The model under review builds one solid part; all positions refer to its coordinate system, in mm. Face numbers are marked on the shaded views. Round coordinates to 2 decimals unless told otherwise and drop trailing zeros. Write each loop counter-clockwise with the first axis right and the second up, starting at its lowest first coordinate (ties: lowest second). Pieces come first, ordered by that corner, then holes. Notation, with made-up numbers: (41.5, -23) -> (54.5, -23) arc R27 cw to (54.5, 16) -> close; hole circle Ø8 at (46, -16.75). An arc over 180 degrees is marked (long way). Return JSON: item names as keys, results as strings. Group by question number.
1. Take a section at B-B, the plane x = 7. Write out the cut boundary in (y, z), then the cut area to 3 significant figures.
2. Mouldability with a two-part tool opening along X and no side actions: class the marked faces 1, 2, 3 and 4 as pulls with the +X half, pulls with the -X half, needs draft (parallel to the pull), parting line crosses it, or undercut.
3. For line 1 along Y through (x, z) = (1.5, 1.15); line 2 along X through (y, z) = (10, 2.6); line 3 along Y through (x, z) = (14, 2.75), list the stretches that pass through material, from the lowest coordinate up. Write a range as from..to.
4. Take a section at A-A, the plane z = 1.35. Write out the cut boundary in (x, y), then the cut area to 3 significant figures.
5. Take a section at D-D, the plane y = -10. Write out the cut boundary in (x, z).
6. Clearance check with flat-ended pins moving along their axes: P1, Ø12, axis at x = 8.5, y = -11, coming from the -Z side; P2, Ø1.5, axis at x = 2, z = 1.5, coming from the -Y side. State where each tip first meets the part, or that it passes through.
7. Take a section at C-C, the plane y = 10. Write out the cut boundary in (x, z).
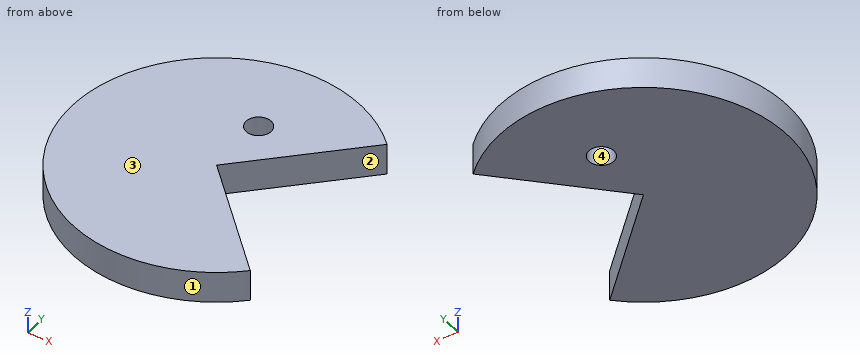
from build123d import *

# Parameters (mm, degrees)
CYLINDER001_R            = 2
CYLINDER001_DEPTH        = 10
CYLINDER_W               = 23
CYLINDER_H               = 5
CYLINDER_ANGLE           = 270
CYLINDER_PLACEMENT_ANGLE = 45


with BuildPart() as obj1:
    # Cylinder001 → Cylinder001 (new body)
    with BuildSketch(Plane(origin=(0, 10, -3), x_dir=(1, 0, 0), z_dir=(0, 0, 1))):
        Circle(CYLINDER001_R)
    extrude(amount=CYLINDER001_DEPTH)


with BuildPart() as obj2:
    # Cylinder → Cylinder (revolve)
    with BuildSketch(Plane.XZ):
        with Locations((11.5, 2.5)):
            Rectangle(CYLINDER_W, CYLINDER_H)
    revolve(axis=Axis((0, 0, 0), (0, 0, 1)), revolution_arc=CYLINDER_ANGLE)


with BuildPart() as obj2_1:
    # Cylinder placement: moved
    add(obj2.part.rotate(Axis((0, 0, 0), (0, 0, 1)), CYLINDER_PLACEMENT_ANGLE))

    # Cut: cut obj1
    add(obj1.part, mode=Mode.SUBTRACT)


solid = obj2_1.part
Output:
{
 "1": {"outline": "(-21.91, 0) -> (-7, 0) -> (-7, 5) -> (-21.91, 5) -> close; (7, 0) -> (21.91, 0) -> (21.91, 5) -> (7, 5) -> close", "area": "149 mm^2"},
 "2": {"face 1": "parting line crosses it", "face 2": "pulls with the +X half", "face 3": "needs draft", "face 4": "undercut"},
 "3": {"line 1": "y = -22.95..-1.5, 1.5..8.68, 11.32..22.95", "line 2": "x = -20.71..-2, 2..10", "line 3": "y = -18.25..-14, 14..18.25"},
 "4": {"outline": "(0, 0) -> (16.26, 16.26) arc R23 ccw (long way) to (16.26, -16.26) -> close; hole circle Ø4 at (0, 10)", "area": "1,230 mm^2"},
 "5": {"outline": "(-20.71, 0) -> (10, 0) -> (10, 5) -> (-20.71, 5) -> close"},
 "6": {"P1": "stops at z = 0", "P2": "stops at y = -22.97"},
 "7": {"outline": "(-20.71, 0) -> (-2, 0) -> (-2, 5) -> (-20.71, 5) -> close; (2, 0) -> (10, 0) -> (10, 5) -> (2, 5) -> close"}
}
